from build123d import *

# Parameters (mm, degrees)
SKETCH1_W             = 203.2
SKETCH1_H             = 152.4
BOSS_EXTRUDE1_DEPTH   = 50.8
SKETCH2_W             = 196.85
SKETCH2_H             = 146.05
CUT_EXTRUDE1_DEPTH    = 47.625
SKETCH4_W             = 228.6
SKETCH4_H             = 177.8
SKETCH4_W_2           = 203.2
SKETCH4_H_2           = 152.4
BOSS_EXTRUDE2_DEPTH   = 6.35
SKETCH7_W             = 212.4456
SKETCH7_H             = 161.6456
SKETCH7_W_2           = 203.2
SKETCH7_H_2           = 152.4
CUT_EXTRUDE2_DEPTH    = 2.6416
F_8_32_TAPPED_HOLE1_D = 3.4544
FILLET3_R             = 4.6228
FILLET4_R             = 9.2456


with BuildPart() as part:
    # Sketch1 → Boss-Extrude1 (new body)
    with BuildSketch(Plane(origin=(0, 0, 0), x_dir=(1, 0, 0), z_dir=(0, 1, 0))):
        Rectangle(SKETCH1_W, SKETCH1_H)
    extrude(amount=BOSS_EXTRUDE1_DEPTH)

    # Sketch2 → Cut-Extrude1 (cut)
    with BuildSketch(Plane(origin=(0, 50.8, 0), x_dir=(1, 0, 0), z_dir=(0, 1, 0))):
        Rectangle(SKETCH2_W, SKETCH2_H)
    extrude(amount=-CUT_EXTRUDE1_DEPTH, mode=Mode.SUBTRACT)

    # Sketch4 → Boss-Extrude2 (add)
    with BuildSketch(Plane(origin=(0, 50.8, 0), x_dir=(1, 0, 0), z_dir=(0, 1, 0))):
        Rectangle(SKETCH4_W, SKETCH4_H)
        Rectangle(SKETCH4_W_2, SKETCH4_H_2, mode=Mode.SUBTRACT)
    extrude(amount=-BOSS_EXTRUDE2_DEPTH)

    # Sketch7 → Cut-Extrude2 (cut)
    with BuildSketch(Plane(origin=(0, 50.8, 0), x_dir=(1, 0, 0), z_dir=(0, 1, 0))):
        Rectangle(SKETCH7_W, SKETCH7_H)
        Rectangle(SKETCH7_W_2, SKETCH7_H_2, mode=Mode.SUBTRACT)
    extrude(amount=-CUT_EXTRUDE2_DEPTH, mode=Mode.SUBTRACT)

    # #8-32 Tapped Hole1 (through all)
    with Locations(Plane(origin=(0, 50.8, 0), x_dir=(1, 0, 0), z_dir=(0, 1, 0))):
        with Locations((55.1307, 84.8614), (110.2614, 84.8614), (110.2614, 28.287133333), (0, 84.8614), (110.2614, -28.287133333), (110.2614, -84.8614), (55.1307, -84.8614), (0, -84.8614), (-55.1307, -84.8614), (-110.2614, -84.8614), (-110.2614, -28.287133333), (-110.2614, 28.287133333), (-110.2614, 84.8614), (-55.1307, 84.8614)):
            Hole(F_8_32_TAPPED_HOLE1_D / 2)

    # Fillet3
    fillet3_edges = [part.edges().sort_by_distance(p)[0] for p in [
        (-101.6, 49.4792, -76.2),
        (101.6, 49.4792, -76.2),
        (101.6, 49.4792, 76.2),
        (-101.6, 49.4792, 76.2),
    ]]
    fillet(fillet3_edges, radius=FILLET3_R)

    # Fillet4
    fillet4_edges = [part.edges().sort_by_distance(p)[0] for p in [
        (-106.2228, 49.4792, -80.8228),
        (106.2228, 49.4792, -80.8228),
        (106.2228, 49.4792, 80.8228),
        (-106.2228, 49.4792, 80.8228),
    ]]
    fillet(fillet4_edges, radius=FILLET4_R)


solid = part.part
The listing builds one solid part. Answer for the finished solid, in the listing's coordinates (mm). A direction names the side the tool comes from. Coordinates: 2 decimals unless noted, no trailing zeros. Order: outer loops, then holes, each group sorted by start corner. A loop starts at its lowest first (then second) coordinate and runs counter-clockwise, first axis right, second up.
Q1. Which of the six approach directions +Z, -Z, +X, -X, +Y, -Y give full straight-line access (tool end or side, diameter ignored) to faces 5 (the face through (-9, 50.8, 85)), 6 (the face through (-1, 22, -76.2)), 7 (the face through (-1, 3.175, -1))?
Q2. A cutting plane is placed at B-B, the plane x = 34. Write down the section's boundary in (y, z) (3 decimals), and give its area (3 significant figures).
Q3. A cutting plane is placed at A-A, the plane y = 6. Write down the section's boundary in (x, z) (3 decimals).
Q4. Given P1, Ø14.5, axis at y = 29, z = 12.5, coming from the +X side; P2, Ø8, axis at y = 11.5, z = -7.5, coming from the -X side; P3, Ø2, axis at x = -90, z = -14.5, coming from the +Y side (3 decimals), each flat-ended and moving along its own axis, determine where each tip first touches the part or whether it passes through.
Q5. For a pull along X with two mould halves and no side action, classify faces 1 (the face through (-114.3, 48, 1)), 2 (the face through (0, 50.8, -74)), 3 (the face through (-103.59, 49.46, 78.04)), 4 (the face through (103.44, 49.46, -78.19)) as pulls with the +X half, pulls with the -X half, needs draft (parallel to the pull), parting line crosses it, or undercut.
Q6. A cutting plane is placed at C-C, the plane z = -23. Write down the section's boundary in (x, y) (3 decimals), and give its area (3 significant figures).
Q7. Consider line 1 (Z direction, x = -37, y = 11) (3 decimals); line 2 (X direction, y = 7, z = 62) (3 decimals); line 3 (Z direction, x = -96.5, y = 44.5) (3 decimals). Determine where each line is inside the solid, lowest interval first.
Answers follow:
1. face 5: +Z, -Z, +X, -X, +Y
1. face 6: -Z, +X, -X, -Y
1. face 7: +Y
2. outline: (0, -76.2) - (44.45, -76.2) - (44.45, -88.9) - (50.8, -88.9) - (50.8, -80.823) - (48.158, -80.823) - (48.158, -76.2) - (50.8, -76.2) - (50.8, -73.025) - (3.175, -73.025) - (3.175, 73.025) - (50.8, 73.025) - (50.8, 76.2) - (48.158, 76.2) - (48.158, 80.823) - (50.8, 80.823) - (50.8, 88.9) - (44.45, 88.9) - (44.45, 76.2) - (0, 76.2) - close
2. area: 923 mm2
3. outline: (-101.6, -76.2) - (101.6, -76.2) - (101.6, 76.2) - (-101.6, 76.2) - close; hole (-98.425, -73.025) - (98.425, -73.025) - (98.425, 73.025) - (-98.425, 73.025) - close
4. P1: stops at x = 101.6
4. P2: stops at x = -101.6
4. P3: stops at y = 3.175
5. face 1: pulls with the -X half
5. face 2: needs draft
5. face 3: undercut
5. face 4: undercut
6. outline: (-114.3, 44.45) - (-101.6, 44.45) - (-101.6, 0) - (101.6, 0) - (101.6, 44.45) - (114.3, 44.45) - (114.3, 50.8) - (106.223, 50.8) - (106.223, 48.158) - (101.6, 48.158) - (101.6, 50.8) - (98.425, 50.8) - (98.425, 3.175) - (-98.425, 3.175) - (-98.425, 50.8) - (-101.6, 50.8) - (-101.6, 48.158) - (-106.223, 48.158) - (-106.223, 50.8) - (-114.3, 50.8) - close
6. area: 1,080 mm2
7. line 1: z = -76.2 to -73.025, 73.025 to 76.2
7. line 2: x = -101.6 to -98.425, 98.425 to 101.6
7. line 3: z = -88.9 to -73.025, 73.025 to 88.9
